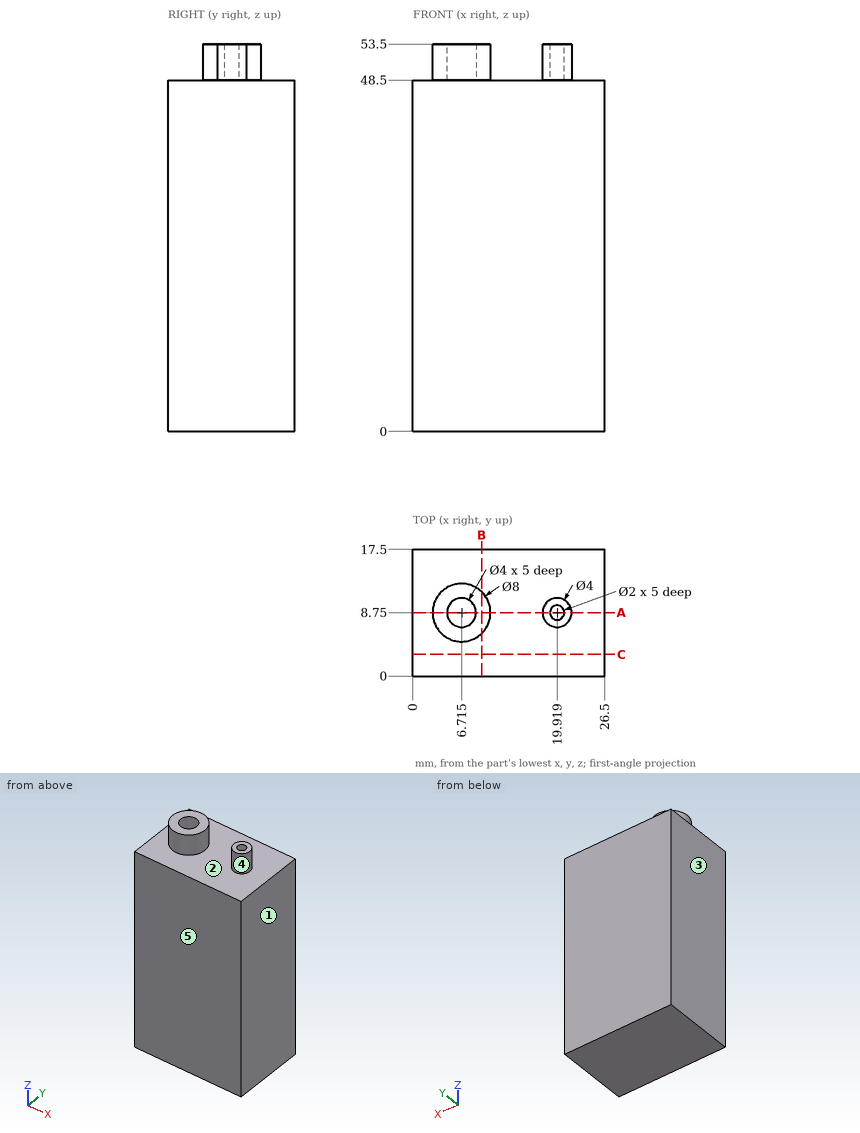
Geometry check sheet. Reference: drawing and pictorial views, mm from the part's lowest x, y, z. A direction names the side the tool comes from. Give positions to 0.01 mm unless a question says otherwise; leave off trailing zeros. Write each loop counter-clockwise with the first axis right and the second up, starting at its lowest first coordinate (ties: lowest second). Pieces come first, ordered by that corner, then holes. Notation, with made-up numbers: M 4,-27 L 38,-27 A20 ccw 38,3 Z; hole C 83.25,-22.5 d10. An arc over 180 degrees is marked long. Answer as CSV lines item,"result". Start each with the question number.
Q1. Section check A-A, the plane y = 8.75. Record the cut outline in (x, z) (3 decimals), then the cut area to 3 significant figures.
Q2. Material ranges on L1, parallel to X at y = 8.5, z = 51.5 (1 decimal); L2, parallel to Z at x = 18, y = 2, recorded low to high.
Q3. Tool access check on the marked faces 1 and 2. Record the directions out of +Z, -Z, +X, -X, +Y, -Y that give a thin tool (end or side, any length) a straight path to the whole face; none if there is none.
Q4. Section check C-C, the plane y = 3. Record the cut outline in (x, z).
Q5. Release check for a two-part mould opening along X. For the marked faces 3, 4 and 5 record: pulls with the +X half, pulls with the -X half, needs draft (parallel to the pull), parting line crosses it, or undercut.
Q6. Section check B-B, the plane x = 9.5. Record the cut outline in (y, z), then the cut area to 3 significant figures.
Q7. Go/stop test with flat-tipped pins: pin 1 (8 mm diameter, centred on x = 21.5, y = 9.5, fed in from -Z); pin 2 (1.8 mm diameter, centred on x = 19.92, y = 8.75, fed in from +Z). Record where each tip stops, or that it passes through.
Geometry says:
1,outline,"M 0,0 L 26.5,0 L 26.5,48.5 L 21.919,48.5 L 21.919,53.5 L 20.919,53.5 L 20.919,48.5 L 18.919,48.5 L 18.919,53.5 L 17.919,53.5 L 17.919,48.5 L 10.715,48.5 L 10.715,53.5 L 8.715,53.5 L 8.715,48.5 L 4.715,48.5 L 4.715,53.5 L 2.715,53.5 L 2.715,48.5 L 0,48.5 Z"
1,area,"1,320 mm^2"
2,L1,"2.7 to 4.7, 8.7 to 10.7, 17.9 to 19, 20.9 to 21.9"
2,L2,"0 to 48.5"
3,face 1,"+Z, -Z, +X, +Y, -Y"
3,face 2,"+Z"
4,outline,"M 0,0 L 26.5,0 L 26.5,48.5 L 0,48.5 Z"
5,face 3,"pulls with the -X half"
5,face 4,"undercut"
5,face 5,"needs draft"
6,outline,"M 0,0 L 17.5,0 L 17.5,48.5 L 11.62,48.5 L 11.62,53.5 L 5.88,53.5 L 5.88,48.5 L 0,48.5 Z"
6,area,"877 mm^2"
7,pin 1,"z = 0"
7,pin 2,"z = 48.5"
